Source: CAD feature listing. Evaluate the final solid. Frame: model axes, mm. A direction names the side the tool comes from. Coordinates: 2 decimals unless noted, no trailing zeros. Order: outer loops, then holes, each group sorted by start corner. A loop starts at its lowest first (then second) coordinate and runs counter-clockwise, first axis right, second up.
```python
from build123d import *

# Parameters (mm, degrees)
F0_W     = 153.4594595432
F0_H     = 88.1393551826
F2_DEPTH = 76.2
F1_R     = 10.1701349395
F1_R_2   = 10.3995540655
F3_DEPTH = 76.201
F5_DEPTH = 101.6
F7_DEPTH = 12.7
F9_DEPTH = 114.301


with BuildPart() as f2:
    # F0 (on Top) → F2 (new body)
    with BuildSketch(Plane.XY):
        Rectangle(F0_W, F0_H)
    extrude(amount=F2_DEPTH)

    # F1 (on face) → F3 (cut, through all)
    with BuildSketch(Plane.XY):
        with Locations((62.4677017331, 0)):
            Circle(F1_R)
        with Locations((-63.608661294, 0)):
            Circle(F1_R_2)
    extrude(amount=F3_DEPTH, mode=Mode.SUBTRACT)

    # F4 (on face) → F5 (join)
    with BuildSketch(Plane.XZ.offset(44.0696775913)):
        with BuildLine():
            ThreePointArc((-35.6539782969, 76.2), (0, 40.5460217031), (35.6539782969, 76.2))
            Line((35.6539782969, 76.2), (-35.6539782969, 76.2))
        make_face()
    extrude(amount=-F5_DEPTH)

    # F6 (on face) → F7 (join)
    with BuildSketch(Plane.XZ.offset(44.0696775913)):
        with BuildLine():
            ThreePointArc((-35.6539782969, 76.2), (0, 40.5460217031), (35.6539782969, 76.2))
            Line((35.6539782969, 76.2), (-35.6539782969, 76.2))
        make_face()
    extrude(amount=F7_DEPTH)

    # F8 (on face) → F9 (cut, through all)
    with BuildSketch(Plane.XZ.offset(56.7696775913)):
        with BuildLine():
            ThreePointArc((-19.8833374867, 76.2), (0, 56.3166625133), (19.8833374867, 76.2))
            Line((19.8833374867, 76.2), (-19.8833374867, 76.2))
        make_face()
        with BuildLine():
            Line((-19.8833374867, 76.2), (19.8833374867, 76.2))
            ThreePointArc((19.8833374867, 76.2), (0, 96.0833374867), (-19.8833374867, 76.2))
        make_face()
    extrude(amount=-F9_DEPTH, mode=Mode.SUBTRACT)


solid = f2.part
```
1. Section query B-B, the plane y = 0. Output: boundary loops of the cut face in (x, z).
2. Material intervals for line 1 along X through (y, z) = (0, 36.5); line 2 along X through (y, z) = (1, 61); line 3 along Y through (x, z) = (-66, 4), sorted ascending.
3. Section query C-C, the plane x = 0. Output: boundary loops of the cut face in (y, z).
4. Section query D-D, the plane z = 38. Output: boundary loops of the cut face in (x, y).
5. Draft query along Y for faces 4 (the flat face through (-1, 44.07, 29)), 5 (the flat face through (-1, -44.07, 30)), 6 (the cylindrical face through (72.17, 3.05, 37.57)), 7 (the flat face through (-76.73, -1, 38)). Return one class per face: +Y half, -Y half, draft (parallel to the pull), parting line (faces both ways), or undercut.
6. Section query A-A, the plane z = 63. Output: boundary loops of the cut face in (x, y), plus the area to 3 significant figures.
7. Access query for faces 1 (the cylindrical face through (-0.784, 50.706, 40.555)), 2 (the flat face through (0, -56.77, 55)), 3 (the cylindrical face through (-0.784, -50.331, 40.555)). Directions: +Z, -Z, +X, -X, +Y, -Y. A direction counts if a zero-diameter tool reaches every point of the face in a straight line with its end or side. Return the directions, or none.
8. Contact query for flat-ended pins moving along their axis: P1, Ø8, axis at x = -3, z = 25.5, coming from the -Y side; P2, Ø23, axis at x = 28, z = 27, coming from the +Y side. Output: stop coordinate, or through.
Answer key:
1. outline: (-76.73, 0) - (-74.01, 0) - (-74.01, 76.2) - (-76.73, 76.2) - close; (-53.21, 0) - (52.3, 0) - (52.3, 76.2) - (19.88, 76.2) arc R19.88 cw to (-19.88, 76.2) - (-53.21, 76.2) - close; (72.64, 0) - (76.73, 0) - (76.73, 76.2) - (72.64, 76.2) - close
2. line 1: x = -76.73 to -74.01, -53.21 to 52.3, 72.64 to 76.73
2. line 2: x = -76.73 to -73.96, -53.26 to -12.82, 12.82 to 52.35, 72.59 to 76.73
2. line 3: y = -44.07 to -10.12, 10.12 to 44.07
3. outline: (-56.77, 40.55) - (-44.07, 40.55) - (-44.07, 0) - (44.07, 0) - (44.07, 40.55) - (57.53, 40.55) - (57.53, 56.32) - (-56.77, 56.32) - close
4. outline: (-76.73, -44.07) - (76.73, -44.07) - (76.73, 44.07) - (-76.73, 44.07) - close; hole circle Ø20.8 at (-63.61, 0); hole circle Ø20.34 at (62.47, 0)
5. face 4: +Y half
5. face 5: -Y half
5. face 6: undercut
5. face 7: draft
6. outline: (-76.73, -44.07) - (-33.12, -44.07) - (-33.12, -56.77) - (-14.87, -56.77) - (-14.87, 57.53) - (-33.12, 57.53) - (-33.12, 44.07) - (-76.73, 44.07) - close; (14.87, -56.77) - (33.12, -56.77) - (33.12, -44.07) - (76.73, -44.07) - (76.73, 44.07) - (33.12, 44.07) - (33.12, 57.53) - (14.87, 57.53) - close; hole circle Ø20.8 at (-63.61, 0); hole circle Ø20.34 at (62.47, 0)
6. area: 11,200 mm2
7. face 1: -Z, +Y
7. face 2: +Z, -Z, +X, -X, -Y
7. face 3: -Z, -Y
8. P1: stops at y = -44.07
8. P2: stops at y = 44.07
